```python
from build123d import *

# Parameters (mm, degrees)
SKETCH_1_R               = 9
EXTRUDE_1_DEPTH          = 3.2
CUT_EXTRUDE_2_REACH      = 15.124
PATTERN_CIRCULAR_1_COUNT = 8
CUT_EXTRUDE_1_REACH      = 14.951
SKETCH_3_R               = 2
PATTERN_CIRCULAR_2_COUNT = 4


with BuildPart() as part:
    # 草图1 → 凸台-拉伸1 (new body)
    with BuildSketch(Plane(origin=(0, 0, 0), x_dir=(1, 0, 0), z_dir=(0, 1, 0))):
        with Locations(Location((0, 0, 0), (0, 0, 270))):
            Circle(SKETCH_1_R)
        with BuildLine():
            Line((-1.058300524, 1.2), (1.058300524, 1.2))
            ThreePointArc((1.058300524, 1.2), (0, -1.6), (-1.058300524, 1.2))
        make_face(mode=Mode.SUBTRACT)
    extrude(amount=EXTRUDE_1_DEPTH)

    # 草图4 → 切除-拉伸2 (cut, up to next)
    with BuildSketch(Plane(origin=(0, 3.2, 0), x_dir=(1, 0, 0), z_dir=(0, 1, 0)), mode=Mode.PRIVATE) as cut_extrude_2_sk1:
        with BuildLine():
            Line((-1.5, 8.874119675), (-0.599498979, 8.19962448))
            ThreePointArc((-0.599498979, 8.19962448), (0, 8), (0.599498979, 8.19962448))
            Line((0.599498979, 8.19962448), (1.5, 8.874119675))
            ThreePointArc((1.5, 8.874119675), (0, 9), (-1.5, 8.874119675))
        make_face()
    cut_extrude_2_tool1 = extrude(cut_extrude_2_sk1.sketch, amount=-CUT_EXTRUDE_2_REACH, mode=Mode.PRIVATE) & part.part
    cut_extrude_2 = cut_extrude_2_tool1.solids().sort_by_distance((0, 3.2, -8.590322))[0]
    add(cut_extrude_2, mode=Mode.SUBTRACT)

    # 阵列(圆周)1: 切除-拉伸2 ×8 about axis
    pattern_circular_1_axis = Axis((0, 0, 0), (0, 1, 0))
    for i in range(1, PATTERN_CIRCULAR_1_COUNT):
        add(cut_extrude_2.rotate(pattern_circular_1_axis, i * 360 / PATTERN_CIRCULAR_1_COUNT), mode=Mode.SUBTRACT)

    # 草图3 → 切除-拉伸1 (cut, up to next)
    with BuildSketch(Plane(origin=(0, 3.2, 0), x_dir=(1, 0, 0), z_dir=(0, 1, 0)), mode=Mode.PRIVATE) as cut_extrude_1_sk1:
        with Locations(Location((0, 5, 0), (0, 0, 270))):
            Circle(SKETCH_3_R)
    cut_extrude_1_tool1 = extrude(cut_extrude_1_sk1.sketch, amount=-CUT_EXTRUDE_1_REACH, mode=Mode.PRIVATE) & part.part
    cut_extrude_1 = cut_extrude_1_tool1.solids().sort_by_distance((0, 3.2, -5))[0]
    add(cut_extrude_1, mode=Mode.SUBTRACT)

    # 阵列(圆周)2: 切除-拉伸1 ×4 about axis
    pattern_circular_2_axis = Axis((0, 0, 0), (0, 1, 0))
    for i in range(1, PATTERN_CIRCULAR_2_COUNT):
        add(cut_extrude_1.rotate(pattern_circular_2_axis, i * 360 / PATTERN_CIRCULAR_2_COUNT), mode=Mode.SUBTRACT)

    # 草图5 → 切除-旋转1 (revolve, cut)
    with BuildSketch(Plane(origin=(0, 0, 0), x_dir=(0, 0, -1), z_dir=(1, 0, 0)), mode=Mode.PRIVATE) as cut_revolve_1_sk:
        Polygon((9.374119675, 2.82841307), (6.778765119, 3.2), (9.374119675, 3.2), align=None)
    cut_revolve_1 = revolve(cut_revolve_1_sk.sketch.rotate(Axis((0, 3.2, 0), (0, -1, 0)), 4.181624795), axis=Axis((0, 3.2, 0), (0, -1, 0)), mode=Mode.SUBTRACT)

    # 镜向1: 切除-旋转1 across plane
    add(cut_revolve_1.mirror(Plane.ZX.offset(1.6)), mode=Mode.SUBTRACT)


solid = part.part
```
Geometry: final body of the model. Coordinates: model frame, mm. A direction names the side the tool comes from. Give positions to 0.01 mm unless a question says otherwise; leave off trailing zeros. Loops run counter-clockwise (first coordinate to the right, second up) from the corner with the lowest first, then second, coordinate; pieces in that order, holes last. Notation, with made-up numbers: (77, -7.75) -> (99, -7.75) arc R17 cw to (99, 9.25) -> close; hole circle Ø7 at (55, 48). An arc over 180 degrees is marked (long way). Return JSON: item names as keys, results as strings.
Item 1: Line query: line 1 (Z direction, x = 0.25, y = 0.45); line 2 (X direction, y = 0.7, z = -5); line 3 (Z direction, x = -6, y = 2.55). Output: solid intervals per line, ascending.
Filled in:
{"line 1": "-8.03 to -6.98, -3.02 to -1.2, 1.58 to 3.02, 6.98 to 8.03", "line 2": "-7.48 to -2, 2 to 7.48", "line 3": "-5.43 to -1.73, 1.73 to 5.43"}
Item 2: Section C-C, the plane x = 0. Output: boundary loops of the cut face in (y, z), plus the area to 3 significant figures.
Filled in:
{"outline": "(0, -3) -> (3.2, -3) -> (3.2, -1.2) -> (0, -1.2) -> close; (0, 1.6) -> (3.2, 1.6) -> (3.2, 3) -> (0, 3) -> close; (0.03, -7) -> (0.17, -8) -> (3.03, -8) -> (3.17, -7) -> close; (0.03, 7) -> (3.17, 7) -> (3.03, 8) -> (0.17, 8) -> close", "area": "16.2 mm^2"}
Item 3: Section B-B, the plane z = 0. Output: boundary loops of the cut face in (x, y).
Filled in:
{"outline": "(-8, 0.17) -> (-7, 0.03) -> (-7, 3.17) -> (-8, 3.03) -> close; (-3, 0) -> (-1.6, 0) -> (-1.6, 3.2) -> (-3, 3.2) -> close; (1.6, 0) -> (3, 0) -> (3, 3.2) -> (1.6, 3.2) -> close; (7, 0.03) -> (8, 0.17) -> (8, 3.03) -> (7, 3.17) -> close"}
Item 4: Section A-A, the plane y = 1.5. Count the separate pieces of the cut face and the enclosed holes in it, plus the area to 3 significant figures.
Filled in:
{"separate pieces": "1", "enclosed holes": "5", "area": "182 mm^2"}
Item 5: Pin query (flat end, axial travel): P1, Ø1.1, axis at x = 0, y = 1, coming from the +Z side. Return the tip coordinate at first contact, or that it passes through.
Filled in:
{"P1": "z = 8.16"}
Item 6: Access query for faces 4 (the flat face through (8.542, 1.62, -1.056)), 5 (the cylindrical face through (-5.663, 1.62, -5.651)). Directions: +Z, -Z, +X, -X, +Y, -Y. A direction counts if a zero-diameter tool reaches every point of the face in a straight line with its end or side. Return the directions, or none.
Filled in:
{"face 4": "+X, +Y, -Y", "face 5": "-Z, -X, +Y, -Y"}
Item 7: Mould query, pull axis Z, two halves, no side actions, for faces 1 (the cylindrical face through (5.651, 1.62, -5.663)), 2 (the flat face through (1.056, 1.62, 8.542)), 3 (the cylindrical face through (8, 2, 0)). Classes: released by +Z, released by -Z, zero draft, split by the parting line, or undercut.
Filled in:
{"face 1": "released by -Z", "face 2": "released by +Z", "face 3": "undercut"}
